Build history of the part. All positions in model axes, mm. A direction names the side the tool comes from. Round coordinates to 2 decimals unless told otherwise and drop trailing zeros. Write each loop counter-clockwise with the first axis right and the second up, starting at its lowest first coordinate (ties: lowest second). Pieces come first, ordered by that corner, then holes.
1) Which spindle directions (+Z, -Z, +X, -X, +Y, -Y) get a long thin tool onto all of the face, cutting with end or side? Do faces 5 (the flat face through (0, -17, 45)), 6 (the flat face through (4, -7, 40)), 7 (the flat face through (2, 19, 30)). Say none if no direction does.
2) Saw through at B-B (x = 4.5). Write the cut outline in (y, z), plus the area to 3 significant figures.
3) Wall check: probe 1 along Y at (x, z) = (11, 10); probe 2 along Y at (x, z) = (-7, 36.5). Give the ranges that are in metal, low to high.
4) Saw through at C-C (z = 15). Write the cut outline in (x, y).
5) Saw through at A-A (y = 16). Write the cut outline in (x, z).
6) Saw through at D-D (y = -14.5). Write the cut outline in (x, z), plus the area to 3 significant figures.
7) Flat gauge pins, fed straight in: pin 1 (22 mm diameter, centred on x = 4, z = 42.5, fed in from +Y); pin 2 (17 mm diameter, centred on x = 3, y = -3.5, fed in from -Z); pin 3 (1.5 mm diameter, centred on x = 6, y = 18.5, fed in from +Z); pin 4 (3.5 mm diameter, centred on x = -15, z = 46, fed in from +Y). Where does each tip first touch, or does it go through?
8) Pull direction X, two halves, no side cores. Call faces 1 (the flat face through (0, -17, 15)), 2 (the flat face through (9, 19, 20)), 3 (the flat face through (0, -20, 20)), 4 (the flat face through (-20, 0, 20)): +X half, -X half, draft (parallel to the pull), parting line (faces both ways), or undercut.
Autodesk Inventor part; units mm, degrees
ref_plane "YZ Plane" through (0, 0, 0) normal (1, 0, 0) x (0, 1, 0)
ref_plane "XZ Plane" through (0, 0, 0) normal (0, 1, 0) x (-1, 0, 0)
ref_plane "XY Plane" through (0, 0, 0) normal (0, 0, 1) x (1, 0, 0)
sketch "スケッチ1" plane through (0, 0, 0) normal (0, 0, 1) x (1, 0, 0)
  line L0 (-17, 17) -> (17, 17)
  line L1 (17, 17) -> (17, -17)
  line L2 (17, -17) -> (-17, -17)
  line L3 (-17, -17) -> (-17, 17)
  line L4 (-17, 17) -> (17, -17) construction
  line L5 (17, 17) -> (-17, -17) construction
  line L6 (-20, 20) -> (20, 20)
  line L7 (20, 20) -> (20, -20)
  line L8 (20, -20) -> (-20, -20)
  line L9 (-20, -20) -> (-20, 20)
  line L10 (-20, 20) -> (20, -20) construction
  line L11 (20, 20) -> (-20, -20) construction
  point P0 (0, 0)
  dimension "d0" = 34
  dimension "d1" = 34
  dimension "d2" = 40
  dimension "d3" = 40
extrude "押し出し1" add sketch "スケッチ1" along normal blind 40
sketch "スケッチ2" plane through (0, 0, 40) normal (0, 0, 1) x (1, 0, 0)
  line L0 (17, 17) -> (17, -17)
  line L1 (-17, -17) -> (-17, 17)
  line L2 (-17, -17) -> (17, -17)
  line L3 (17, -17) -> (17, -7)
  line L4 (17, -7) -> (-17, -7)
  line L5 (-17, -7) -> (-17, -17)
  line L6 (-17, 17) -> (-10, 17)
  line L7 (-10, 17) -> (-10, -7)
  line L8 (-10, -7) -> (-17, -7)
  line L9 (-17, -7) -> (-17, 17)
  point P0 (0, 0)
  dimension "d6" = 10
  dimension "d7" = 7
extrude "押し出し2" add sketch "スケッチ2" along normal blind 10 and the other way blind 10
sketch "スケッチ3" plane through (-20, 20, 0) normal (0, 1, 0) x (1, 0, 0)
  line L0 (40, -40) -> (37, -40)
  line L1 (37, -40) -> (37, -30)
  line L2 (37, -30) -> (40, -30)
  line L3 (40, -30) -> (40, -40)
  line L4 (37, -40) -> (22, -40)
  line L5 (22, -40) -> (22, -20)
  line L6 (22, -20) -> (37, -20)
  line L7 (37, -20) -> (37, -40)
  point P0 (20, 0)
  dimension "d12" = 3
  dimension "d13" = 10
  dimension "d14" = 15
  dimension "d15" = 20
extrude "押し出し3" cut sketch "スケッチ3" against normal blind 10 contours L4 L5 L6 L7 L1
properties part number "知能ロボコン角材延長"
Evaluation:
1. face 5: +Z, +X, -X, -Y
1. face 6: +Z, -Z
1. face 7: +Z, +Y
2. outline: (-20, 0) - (-17, 0) - (-17, 30) - (-7, 30) - (-7, 50) - (-17, 50) - (-17, 40) - (-20, 40) - close; (17, 0) - (20, 0) - (20, 20) - (17, 20) - close
2. area: 380 mm2
3. probe 1: y = -20 to -17, 17 to 20
3. probe 2: y = -20 to -7, 17 to 20
4. outline: (-20, -20) - (20, -20) - (20, 20) - (-20, 20) - close; hole (-17, -17) - (17, -17) - (17, 17) - (-17, 17) - close
5. outline: (-20, 0) - (-17, 0) - (-17, 30) - (-10, 30) - (-10, 50) - (-17, 50) - (-17, 40) - (-20, 40) - close; (17, 0) - (20, 0) - (20, 40) - (17, 40) - close
6. outline: (-20, 0) - (-17, 0) - (-17, 30) - (17, 30) - (17, 0) - (20, 0) - (20, 40) - (17, 40) - (17, 50) - (-17, 50) - (-17, 40) - (-20, 40) - close
6. area: 920 mm2
7. pin 1: stops at y = 20
7. pin 2: stops at z = 30
7. pin 3: stops at z = 20
7. pin 4: stops at y = 17
8. face 1: undercut
8. face 2: undercut
8. face 3: draft
8. face 4: -X half
